Geometry check sheet. Reference: drawing and pictorial views, mm from the part's lowest x, y, z. A direction names the side the tool comes from. Coordinates: 2 decimals unless noted, no trailing zeros. Write each loop counter-clockwise with the first axis right and the second up, starting at its lowest first coordinate (ties: lowest second). Pieces come first, ordered by that corner, then holes. Notation, with made-up numbers: (-1, 37) - (26, 37) arc R7 ccw to (26, 46) - close; hole circle Ø8 at (76.25, 22.25). An arc over 180 degrees is marked (long way). Answer as CSV lines item,"result". Start each with the question number.
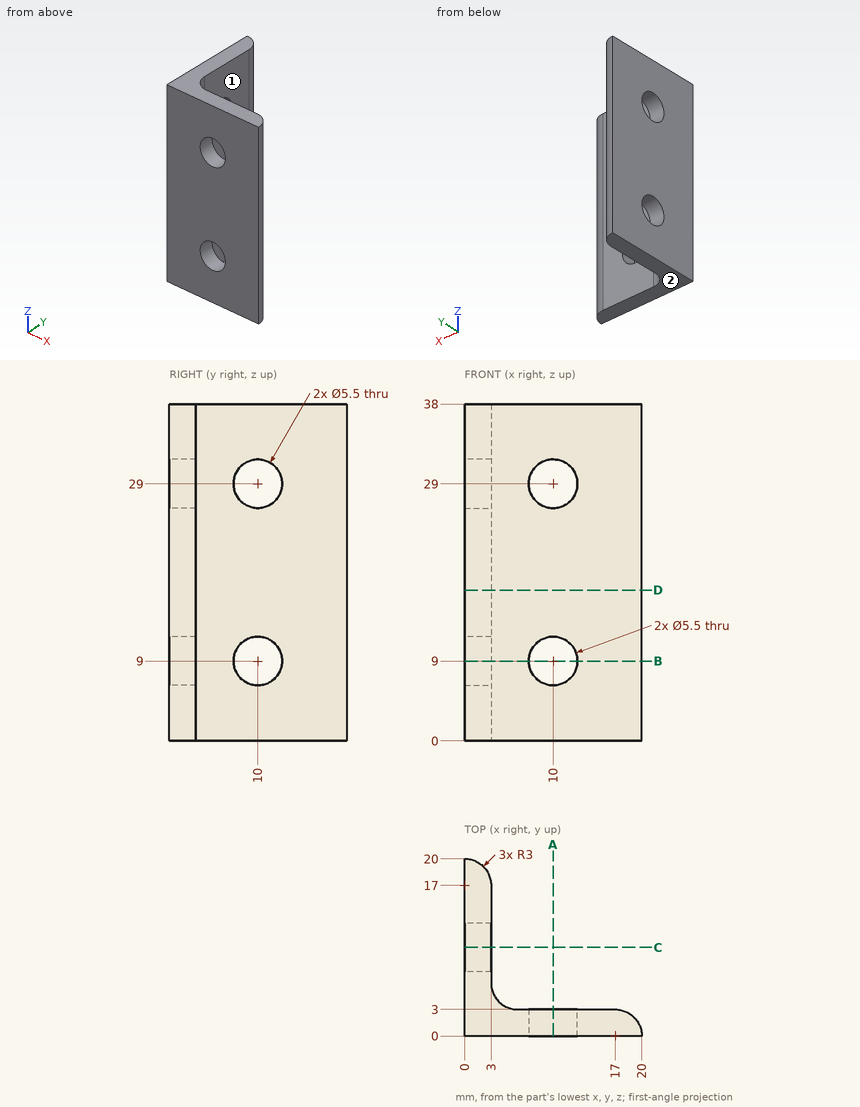
1. Scan lines: line 1 along Z through (x, y) = (1.95, 10); line 2 along Y through (x, z) = (7.5, 35.5). Record each from-to range of solid material in increasing order. Write a range as from..to.
2. Cross-section at B-B (z = 9). Record the cut outline in (x, y).
3. Depth check by flat-ended pin: P1, Ø4.5, axis at y = 10, z = 29, coming from the -X side; P2, Ø2, axis at y = 10.5, z = 34, coming from the +X side; P3, Ø12, axis at x = 11.5, z = 11, coming from the +Y side; P4, Ø6, axis at x = 7, z = 5.5, coming from the +Y side. Enter the tip coordinate at first touch or a pass-through.
4. Access from +Z, -Z, +X, -X, +Y, -Y to the whole of each face (thin tool, end or side, straight path). Record for the marked faces 1 and 2.
5. Cross-section at D-D (z = 17). Record the cut outline in (x, y), and give its area (3 significant figures).
6. Cross-section at A-A (x = 10). Record the cut outline in (y, z).
Completed:
1,line 1,"z = 0..6.25, 11.75..26.25, 31.75..38"
1,line 2,"y = 0..3"
2,outline,"(0, 0) - (7.25, 0) - (7.25, 3) - (6, 3) arc R3 cw to (3, 6) - (3, 7.25) - (0, 7.25) - close; (0, 12.75) - (3, 12.75) - (3, 17) arc R3 ccw to (0, 20) - close; (12.75, 0) - (20, 0) arc R3 ccw to (17, 3) - (12.75, 3) - close"
3,P1,"passes through"
3,P2,"stops at x = 3"
3,P3,"stops at y = 3.04"
3,P4,"stops at y = 3.76"
4,face 1,"+Z, -Z, +X, +Y"
4,face 2,"-Z, +X, -X, +Y, -Y"
5,outline,"(0, 0) - (20, 0) arc R3 ccw to (17, 3) - (6, 3) arc R3 cw to (3, 6) - (3, 17) arc R3 ccw to (0, 20) - close"
5,area,"109 mm2"
6,outline,"(0, 0) - (3, 0) - (3, 6.25) - (0, 6.25) - close; (0, 11.75) - (3, 11.75) - (3, 26.25) - (0, 26.25) - close; (0, 31.75) - (3, 31.75) - (3, 38) - (0, 38) - close"
